Print and shaded views of the part. All mm, measured from the part's lowest x, y and z. Coordinates: 2 decimals unless noted, no trailing zeros. Order: outer loops, then holes, each group sorted by start corner. A loop starts at its lowest first (then second) coordinate and runs counter-clockwise, first axis right, second up. Notation, with made-up numbers: (-17, 27) -> (33, 27) arc R30 cw to (33, 62) -> close; hole circle Ø8 at (89, 86). An arc over 180 degrees is marked (long way). Return JSON: item names as keys, results as strings. Group by question number.
1) Cut at A-A (x = 38.1). Write the cut outline in (y, z) (1 decimal).
2) Cut at B-B (z = 24). Write the cut outline in (x, y) (1 decimal), and give its area (3 significant figures).
3) Probe line 1 (Y direction, x = 72, z = 38) (1 decimal); line 2 (X direction, y = 13, z = 39); line 3 (Y direction, x = 38, z = 7) (1 decimal). List the from-to ranges inside material, lowest first.
4) Cut at C-C (y = 6.5). Write the cut outline in (x, z), and give its area (3 significant figures).
5) Flat gauge pins, fed straight in: pin 1 (1.5 mm diameter, centred on x = 18.5, y = 14.5, fed in from +Z); pin 2 (5 mm diameter, centred on x = 38.1, y = 13.76, fed in from +Z); pin 3 (4 mm diameter, centred on y = 31, z = 41.5, fed in from -X); pin 4 (7.5 mm diameter, centred on y = 27.52, z = 38.1, fed in from +X). Where does each tip first touch, or does it go through?
6) Cut at D-D (x = 60.5). Write the cut outline in (y, z) (1 decimal), and give its area (3 significant figures).
7) Pull direction Z, two halves, no side cores. Call the marked faces 1, 2 and 3: +Z half, -Z half, draft (parallel to the pull), parting line (faces both ways), or undercut.
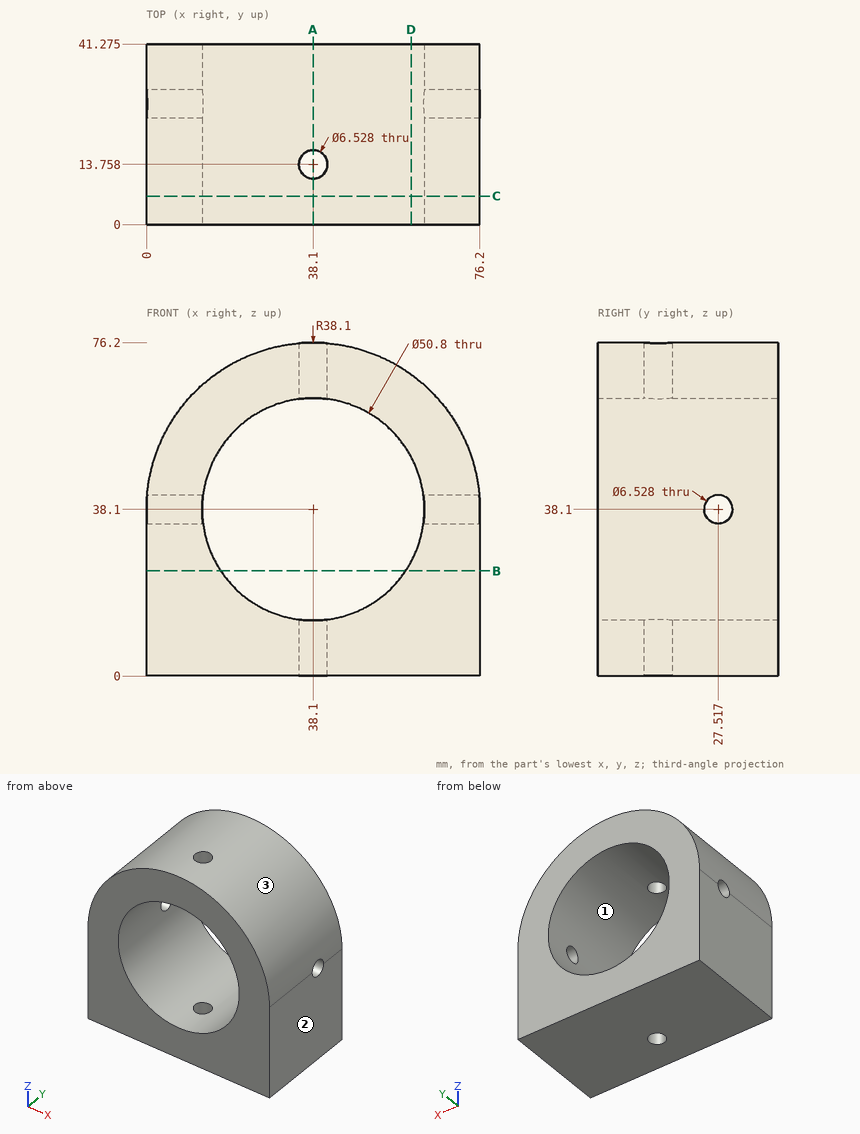
Answers below:
{
 "1": {"outline": "(0, 0) -> (10.5, 0) -> (10.5, 12.7) -> (0, 12.7) -> close; (0, 63.5) -> (10.5, 63.5) -> (10.5, 76.2) -> (0, 76.2) -> close; (17, 0) -> (41.3, 0) -> (41.3, 12.7) -> (17, 12.7) -> close; (17, 63.5) -> (41.3, 63.5) -> (41.3, 76.2) -> (17, 76.2) -> close"},
 "2": {"outline": "(0, 0) -> (17, 0) -> (17, 41.3) -> (0, 41.3) -> close; (59.2, 0) -> (76.2, 0) -> (76.2, 41.3) -> (59.2, 41.3) -> close", "area": "1,400 mm^2"},
 "3": {"line 1": "y = 0 to 24.3, 30.8 to 41.3", "line 2": "x = 0.01 to 12.72, 63.48 to 76.19", "line 3": "y = 0 to 10.5, 17 to 41.3"},
 "4": {"outline": "(0, 0) -> (76.2, 0) -> (76.2, 38.1) arc R38.1 ccw to (0, 38.1) -> close; hole circle Ø50.8 at (38.1, 38.1)", "area": "3,160 mm^2"},
 "5": {"pin 1": "stops at z = 71.21", "pin 2": "passes through", "pin 3": "stops at x = 0.03", "pin 4": "stops at x = 76.2"},
 "6": {"outline": "(0, 0) -> (41.3, 0) -> (41.3, 26.1) -> (0, 26.1) -> close; (0, 50.1) -> (41.3, 50.1) -> (41.3, 68.9) -> (0, 68.9) -> close", "area": "1,860 mm^2"},
 "7": {"face 1": "undercut", "face 2": "draft", "face 3": "+Z half"}
}
